Here's how the part is built. I have some questions about the finished solid (model axes, mm). Face numbers are marked on the shaded views. A direction names the side the tool comes from. Give positions to 0.01 mm unless a question says otherwise; leave off trailing zeros. Order: outer loops, then holes, each group sorted by start corner. A loop starts at its lowest first (then second) coordinate and runs counter-clockwise, first axis right, second up.
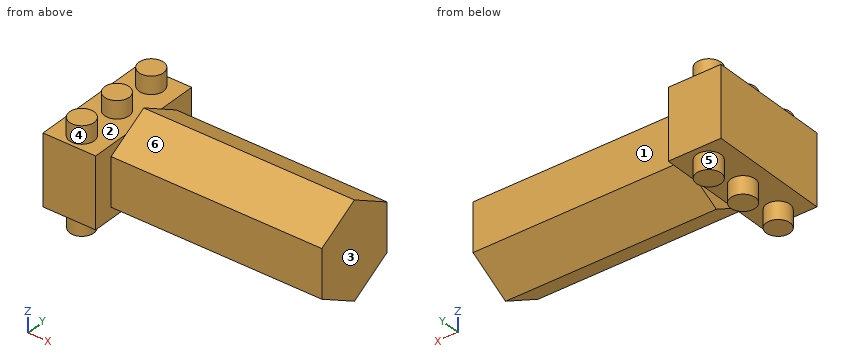
from build123d import *

# Parameters (mm, degrees)
SKETCH2_W           = 7.62
SKETCH2_H           = 17.78
BOSS_EXTRUDE1_DEPTH = 10.16
BOSS_EXTRUDE3_DEPTH = 30.48
SKETCH8_R           = 1.778
SKETCH8_R_2         = 1.721357936
BOSS_EXTRUDE4_DEPTH = 2.54
BOSS_EXTRUDE5_START = 2.54
SKETCH6_R           = 1.778
BOSS_EXTRUDE5_DEPTH = 2.54


with BuildPart() as part:
    # Sketch2 → Boss-Extrude1 (new body)
    with BuildSketch(Plane.XY):
        with Locations((3.81, 8.89)):
            Rectangle(SKETCH2_W, SKETCH2_H)
    extrude(amount=BOSS_EXTRUDE1_DEPTH)

    # Sketch3 → Boss-Extrude3 (add)
    with BuildSketch(Plane(origin=(7.62, 0, 0), x_dir=(0, 0, -1), z_dir=(1, 0, 0))):
        Polygon((1.885696, 8.89), (-1.597152, 14.922469691), (-8.562848, 14.922469691), (-12.045696, 8.89), (-8.562848, 2.857530309), (-1.597152, 2.857530309), align=None)
    extrude(amount=BOSS_EXTRUDE3_DEPTH)

    # Sketch8 → Boss-Extrude4 (add)
    with BuildSketch(Plane(origin=(0, 0, 0), x_dir=(-1, 0, 0), z_dir=(0, 0, -1))):
        with Locations((-3.81, 15.167140335)):
            Circle(SKETCH8_R)
        with Locations((-3.81, 8.817140335)):
            Circle(SKETCH8_R)
        with Locations((-3.81, 2.31394822)):
            Circle(SKETCH8_R_2)
    extrude(amount=BOSS_EXTRUDE4_DEPTH)

    # Sketch6 → Boss-Extrude5 (add)
    with BuildSketch(Plane.XY.offset(10.16).offset(BOSS_EXTRUDE5_START)):
        with Locations(Location((3.81, 15.167140335, 0), (0, 0, 180))):
            Circle(SKETCH6_R)
        with Locations(Location((3.81, 8.817140335, 0), (0, 0, 180))):
            Circle(SKETCH6_R)
        with Locations(Location((3.81, 2.31394822, 0), (0, 0, 180))):
            Circle(SKETCH6_R)
    extrude(amount=-BOSS_EXTRUDE5_DEPTH)


solid = part.part
Q1. For the marked faces 4, 5 and 6, which set-ups out of +Z, -Z, +X, -X, +Y, -Y let a thin tool reach every point of the face, with its end or its side?
Filled sheet:
face 4: +Z
face 5: -Z
face 6: +Z, +X, -Y
Q2. If we section it at D-D on y = 12.75: List the corners of the cut face in (x, z) for me.
Filled sheet:
outline: (0, 0) - (7.62, 0) - (7.62, 0.34) - (38.1, 0.34) - (38.1, 9.82) - (7.62, 9.82) - (7.62, 10.16) - (0, 10.16) - close
Q3. If we section it at B-B on z = 11: List the corners of the cut face in (x, y) for me.
Filled sheet:
outline: circle Ø3.56 at (3.81, 2.31); circle Ø3.56 at (3.81, 8.82); circle Ø3.56 at (3.81, 15.17); (7.62, 7.08) - (38.1, 7.08) - (38.1, 10.7) - (7.62, 10.7) - close
Q4. I need wall thicknesses on L1, parallel to Y at x = 20, z = 4.25; L2, parallel to X at y = 16.5, z = 10; L3, parallel to Y at x = 28.5, z = 0. Which ranges of each line are inside material? Lowest first, please.
Filled sheet:
L1: y = 2.86 to 14.92
L2: x = 0 to 7.62
L3: y = 5.62 to 12.16
Q5. If we section it at C-C on z = 5: List the corners of the cut face in (x, y) for me.
Filled sheet:
outline: (0, 0) - (7.62, 0) - (7.62, 2.86) - (38.1, 2.86) - (38.1, 14.92) - (7.62, 14.92) - (7.62, 17.78) - (0, 17.78) - close
Q6. Thinking about a two-plate mould opening in Y: for the marked faces 1, 2 and 3, which applies, released by +Y, released by -Y, zero draft, split by the parting line, or undercut?
Filled sheet:
face 1: released by +Y
face 2: undercut
face 3: zero draft
Q7. I'm going to push flat-ended pins straight in: P1, Ø1.5, axis at x = 15, z = -1, coming from the -Y side; P2, Ø2, axis at x = 23.5, z = 3.5, coming from the +Y side; P3, Ø10, axis at x = 34, y = 10.5, coming from the +Z side. Where does each tip first touch, or does it pass through?
Filled sheet:
P1: stops at y = 6.06
P2: stops at y = 14.92
P3: stops at z = 12.05
Q8. If we section it at A-A on x = 3.81: List the corners of the cut face in (y, z) for me.
Filled sheet:
outline: (0, 0) - (0.59, 0) - (0.59, -2.54) - (4.04, -2.54) - (4.04, 0) - (7.04, 0) - (7.04, -2.54) - (10.6, -2.54) - (10.6, 0) - (13.39, 0) - (13.39, -2.54) - (16.95, -2.54) - (16.95, 0) - (17.78, 0) - (17.78, 10.16) - (16.95, 10.16) - (16.95, 12.7) - (13.39, 12.7) - (13.39, 10.16) - (10.6, 10.16) - (10.6, 12.7) - (7.04, 12.7) - (7.04, 10.16) - (4.09, 10.16) - (4.09, 12.7) - (0.54, 12.7) - (0.54, 10.16) - (0, 10.16) - close
